Autodesk Inventor part; units mm, degrees
ref_plane "Work Plane1" through (0, 0, 0) normal (0, 0, 1) x (1, 0, 0)
ref_plane "YZ Plane" through (0, 0, 0) normal (1, 0, 0) x (0, 1, 0)
ref_plane "XZ Plane" through (0, 0, 0) normal (0, 1, 0) x (-1, 0, 0)
ref_plane "Work Plane1" through (0, 0, 0) normal (0, 0, 1) x (1, 0, 0)
sketch "Sketch2" plane through (0, 0, 0) normal (0, 0, 1) x (1, 0, 0)
  circle A0 centre (0, 0) radius 16.75
  circle A1 centre (0, 0) radius 50
  point P0 (0, 0)
  dimension "d0" = 33.5
  dimension "d25" = 100
extrude "Extrusion1" add sketch "Sketch2" along normal blind 3
sketch "Sketch3" plane through (0, 0, 0) normal (0, 0, -1) x (-1, 0, 0)
  circle A0 centre (0, 0) radius 24.25
  circle A1 centre (0, 0) radius 21.75
  point P0 (0, 0)
  dimension "d4" = 48.5
  dimension "d26" = 2.5
extrude "Extrusion2" add sketch "Sketch3" along normal blind 300
sketch "Sketch4" plane through (0, 0, 0) normal (0, 0, -1) x (-1, 0, 0)
  circle A0 centre (0, 0) radius 16.75
  circle A1 centre (0, 0) radius 37.5 construction
  circle A2 centre (37.5, 0) radius 3
  circle A3 centre (0, 0) radius 37.5 construction
  circle A4 centre (0, 37.5) radius 3
  circle A5 centre (0, 0) radius 37.5 construction
  circle A6 centre (-37.5, 0) radius 3
  circle A7 centre (0, 0) radius 37.5 construction
  circle A8 centre (0, -37.5) radius 3
  point P0 (0, 0)
  dimension "d9" = 75
  dimension "d10" = 6
  dimension "d13" = 360
hole "Hole1" at (-37.5, 0, 0) at (0, -37.5, 0) at (37.5, 0, 0) at (0, 37.5, 0) direction (0, 0, 1) diameter 6 end through all
properties part number "40mm_flange"
Could you check a few things on this model? Use its own coordinates, in mm. A direction names the side the tool comes from. Coordinates: 2 decimals unless noted, no trailing zeros. Write each loop counter-clockwise with the first axis right and the second up, starting at its lowest first coordinate (ties: lowest second). Pieces come first, ordered by that corner, then holes. Notation, with made-up numbers: (44, 69) -> (99, 69) arc R13 ccw to (99, 89) -> close; hole circle Ø10 at (76, 0). An arc over 180 degrees is marked (long way). Return JSON: item names as keys, results as strings.
(1) Imagine slicing it at D-D, the plane x = -37.5. Please give me the cut outline in (y, z), then the cut area to 3 significant figures.
Numbers:
{"outline": "(-33.07, 0) -> (-3, 0) -> (-3, 3) -> (-33.07, 3) -> close; (3, 0) -> (33.07, 0) -> (33.07, 3) -> (3, 3) -> close", "area": "180 mm2"}
(2) I'm going to push flat-ended pins straight in: pin 1 (5 mm diameter, centred on y = -23.5, z = -133.5, fed in from -X); pin 2 (12 mm diameter, centred on x = -4, z = -140.5, fed in from -Y); pin 3 (6 mm diameter, centred on x = -8, z = -96.5, fed in from +Y); pin 4 (5 mm diameter, centred on x = 37.5, y = 0, fed in from +Z). Where does each tip first touch, or does it pass through?
Numbers:
{"pin 1": "stops at x = -12.13", "pin 2": "stops at y = -24.25", "pin 3": "stops at y = 23.73", "pin 4": "passes through"}
(3) Which directions (+Z, -Z, +X, -X, +Y, -Y) give clear straight access to the entire face, cutting with the end or side of a thin tool? Please do faces 5 (the cylindrical face through (2.831, -21.565, -147.9)), 6 (the cylindrical face through (-40.474, -0.391, 1.521)).
Numbers:
{"face 5": "-Z", "face 6": "+Z, -Z"}
(4) Imagine slicing it at A-A, the plane y = 0. Please give me the cut outline in (x, z), then the cut area to 3 significant figures.
Numbers:
{"outline": "(-50, 0) -> (-40.5, 0) -> (-40.5, 3) -> (-50, 3) -> close; (-34.5, 0) -> (-24.25, 0) -> (-24.25, -300) -> (-21.75, -300) -> (-21.75, 0) -> (-16.75, 0) -> (-16.75, 3) -> (-34.5, 3) -> close; (16.75, 0) -> (21.75, 0) -> (21.75, -300) -> (24.25, -300) -> (24.25, 0) -> (34.5, 0) -> (34.5, 3) -> (16.75, 3) -> close; (40.5, 0) -> (50, 0) -> (50, 3) -> (40.5, 3) -> close", "area": "1,660 mm2"}
(5) Imagine slicing it at C-C, the plane y = -12. Please give me the cut outline in (x, z), then the cut area to 3 significant figures.
Numbers:
{"outline": "(-48.54, 0) -> (-21.07, 0) -> (-21.07, -300) -> (-18.14, -300) -> (-18.14, 0) -> (-11.69, 0) -> (-11.69, 3) -> (-48.54, 3) -> close; (11.69, 0) -> (18.14, 0) -> (18.14, -300) -> (21.07, -300) -> (21.07, 0) -> (48.54, 0) -> (48.54, 3) -> (11.69, 3) -> close", "area": "1,980 mm2"}
(6) I need wall thicknesses on L1, parallel to Y at x = 0, z = 2.4; L2, parallel to Z at x = -1, y = -29.5; L3, parallel to Y at x = 0, z = -182. Which ranges of each line are inside material? Lowest first, please.
Numbers:
{"L1": "y = -50 to -40.5, -34.5 to -16.75, 16.75 to 34.5, 40.5 to 50", "L2": "z = 0 to 3", "L3": "y = -24.25 to -21.75, 21.75 to 24.25"}
(7) We'd pull the mould along X, two halves only. Please class faces 1 (the cylindrical face through (-11.19, 21.514, -147.9)), 2 (the flat face through (-1, -22, 3)), 3 (the cylindrical face through (-3.63, 16.35, 1.48)), 4 (the cylindrical face through (-0.1, 34.5, 1.5)): +X half, -X half, draft (parallel to the pull), parting line (faces both ways), or undercut.
Numbers:
{"face 1": "parting line", "face 2": "draft", "face 3": "undercut", "face 4": "undercut"}
